```python
from build123d import *

# Parameters (mm, degrees)
SKETCH1_W                                        = 109
SKETCH1_H                                        = 140
BOSS_EXTRUDE1_DEPTH                              = 4
CBORE_FOR_M4_PAN_HEAD_MACHINE_SCREW1_D           = 4.5
CBORE_FOR_M4_PAN_HEAD_MACHINE_SCREW1_CBORE_D     = 9
CBORE_FOR_M4_PAN_HEAD_MACHINE_SCREW1_CBORE_DEPTH = 3.1
SKETCH6_W                                        = 25.091702427
SKETCH6_H                                        = 69.60512686
CUT_EXTRUDE1_DEPTH                               = 89.804560694
SKETCH7_W                                        = 140
SKETCH7_H                                        = 35
BOSS_EXTRUDE2_DEPTH                              = 4
FILLET1_R                                        = 10
BOSS_EXTRUDE3_DEPTH                              = 15
SKETCH9_W                                        = 2
SKETCH9_H                                        = 35
BOSS_EXTRUDE4_DEPTH                              = 140
CUT_EXTRUDE3_DEPTH                               = 101.444014257
SKETCH11_W                                       = 109
SKETCH11_H                                       = 15
CUT_EXTRUDE4_DEPTH                               = 2
FILLET6_R                                        = 5
CUT_EXTRUDE5_REACH                               = 103.198
SKETCH13_W                                       = 4
SKETCH13_H                                       = 73.569558417
CUT_EXTRUDE5_DIRECTION_2_REACH                   = 103.198
SKETCH14_W                                       = 4
SKETCH14_H                                       = 10
BOSS_EXTRUDE5_DEPTH                              = 38.816595147
FILLET9_R                                        = 2.5


with BuildPart() as part:
    # Sketch1 → Boss-Extrude1 (new body)
    with BuildSketch(Plane.XY):
        Rectangle(SKETCH1_W, SKETCH1_H)
    extrude(amount=BOSS_EXTRUDE1_DEPTH)

    # CBORE for M4 Pan Head Machine Screw1 (through all)
    with Locations(Plane.XY.offset(4)):
        with Locations((-19.408297573, 58.521958499), (19.408297573, 58.521958499), (-44.361823025, -9.60512686), (44.559866877, -9.60512686)):
            CounterBoreHole(CBORE_FOR_M4_PAN_HEAD_MACHINE_SCREW1_D / 2, CBORE_FOR_M4_PAN_HEAD_MACHINE_SCREW1_CBORE_D / 2, CBORE_FOR_M4_PAN_HEAD_MACHINE_SCREW1_CBORE_DEPTH)

    # Sketch6 → Cut-Extrude1 (cut, through all)
    with BuildSketch(Plane.XY.offset(4)):
        with Locations((-41.954148786, 35.19743657)):
            Rectangle(SKETCH6_W, SKETCH6_H)
        with Locations((41.954148786, 35.19743657)):
            Rectangle(SKETCH6_W, SKETCH6_H)
    extrude(amount=-CUT_EXTRUDE1_DEPTH, mode=Mode.SUBTRACT)

    # Sketch7 → Boss-Extrude2 (add, through all)
    with BuildSketch(Plane.XY.offset(4)):
        with Locations((0, -52.5)):
            Rectangle(SKETCH7_W, SKETCH7_H)
    extrude(amount=-BOSS_EXTRUDE2_DEPTH)

    # Fillet1
    fillet1_edges = [part.edges().sort_by_distance(p)[0] for p in [
        (-29.408297573, 70, 2),
        (-54.5, 0.39487314, 2),
        (29.408297573, 70, 2),
        (54.5, 0.39487314, 2),
    ]]
    fillet(fillet1_edges, radius=FILLET1_R)

    # Sketch8 → Boss-Extrude3 (add)
    with BuildSketch(Plane.XY.offset(4)):
        Polygon((-70, -35), (-70, -70), (70, -70), (70, -35), (68, -35), (68, -68), (-68, -68), (-68, -35), align=None)
    extrude(amount=BOSS_EXTRUDE3_DEPTH)

    # Sketch9 → Boss-Extrude4 (add, through all)
    with BuildSketch(Plane.ZY.offset(70)):
        with Locations((20, -52.5)):
            Rectangle(SKETCH9_W, SKETCH9_H)
    extrude(amount=-BOSS_EXTRUDE4_DEPTH)

    # Sketch10 → Cut-Extrude3 (cut, through all)
    with BuildSketch(Plane.XY.offset(4)):
        Polygon((-19.408297573, 48.521958499), (-9.408297573, 48.521958499), (-9.408297573, 60), (9.408297573, 60), (9.408297573, 48.521958499), (19.408297573, 48.521958499), (19.408297573, -9.60512686), (34.559866877, -9.60512686), (34.559866877, -19.60512686), (44.5, -19.60512686), (44.5, -60), (-44.5, -60), (-44.5, -19.60512686), (-34.361823025, -19.60512686), (-34.361823025, -9.60512686), (-19.408297573, -9.60512686), align=None)
    extrude(amount=-CUT_EXTRUDE3_DEPTH, mode=Mode.SUBTRACT)

    # Sketch11 → Cut-Extrude4 (cut)
    with BuildSketch(Plane.XY.offset(21)):
        with Locations((0, -42.5)):
            Rectangle(SKETCH11_W, SKETCH11_H)
    extrude(amount=-CUT_EXTRUDE4_DEPTH, mode=Mode.SUBTRACT)

    # Fillet6
    fillet6_edges = [part.edges().sort_by_distance(p)[0] for p in [
        (-54.5, -50, 20),
        (54.5, -50, 20),
        (54.5, -35, 20),
        (-54.5, -35, 20),
    ]]
    fillet(fillet6_edges, radius=FILLET6_R)

    # Cut-Extrude5: up to this face of the body (flat: up to its plane)
    cut_extrude5_end = Plane(part.part.faces().sort_by_distance((-29.408297573, 30.19743657, 2))[0])
    # Sketch13 → Cut-Extrude5 (cut, up to the picked face)
    with BuildSketch(Plane(origin=(0, 0, 0), x_dir=(0, 0, -1), z_dir=(1, 0, 0)), mode=Mode.PRIVATE) as cut_extrude5_sk1:
        with Locations((-2, 37.179652349)):
            Rectangle(SKETCH13_W, SKETCH13_H)
    cut_extrude5_tool1 = split(extrude(cut_extrude5_sk1.sketch, amount=-CUT_EXTRUDE5_REACH, mode=Mode.PRIVATE), bisect_by=cut_extrude5_end, keep=Keep.BOTH, mode=Mode.PRIVATE)
    add(cut_extrude5_tool1.solids().sort_by(Axis((0, 37.179652, 2), (-1, 0, 0)))[0], mode=Mode.SUBTRACT)

    # Cut-Extrude5 direction 2: up to this face of the body (flat: up to its plane)
    cut_extrude5_direction_2_end = Plane(part.part.faces().sort_by_distance((29.408297573, 30.19743657, 2))[0])
    # Sketch13 → Cut-Extrude5 direction 2 (cut, up to the picked face)
    with BuildSketch(Plane(origin=(0, 0, 0), x_dir=(0, 0, -1), z_dir=(1, 0, 0)), mode=Mode.PRIVATE) as cut_extrude5_direction_2_sk1:
        with Locations((-2, 37.179652349)):
            Rectangle(SKETCH13_W, SKETCH13_H)
    cut_extrude5_direction_2_tool1 = split(extrude(cut_extrude5_direction_2_sk1.sketch, amount=CUT_EXTRUDE5_DIRECTION_2_REACH, mode=Mode.PRIVATE), bisect_by=cut_extrude5_direction_2_end, keep=Keep.BOTH, mode=Mode.PRIVATE)
    add(cut_extrude5_direction_2_tool1.solids().sort_by(Axis((0, 37.179652, 2), (1, 0, 0)))[0], mode=Mode.SUBTRACT)

    # Sketch14 → Boss-Extrude5 (add)
    with BuildSketch(Plane.ZY.offset(-19.408297573)):
        with Locations((2, -4.60512686)):
            Rectangle(SKETCH14_W, SKETCH14_H)
    extrude(amount=BOSS_EXTRUDE5_DEPTH)

    # Fillet9
    fillet9_edges = [part.edges().sort_by_distance(p)[0] for p in [
        (34.559866877, -9.60512686, 2),
        (34.559866877, -19.60512686, 2),
        (44.5, -19.60512686, 2),
        (44.5, -60, 2),
        (-44.5, -60, 2),
        (-44.5, -19.60512686, 2),
        (-34.361823025, -19.60512686, 2),
        (-34.361823025, -9.60512686, 2),
    ]]
    fillet(fillet9_edges, radius=FILLET9_R)


solid = part.part
```
Model file for the job. Use its own axes, mm. A direction names the side the tool comes from. Coordinates: 2 decimals unless noted, no trailing zeros. Write each loop counter-clockwise with the first axis right and the second up, starting at its lowest first coordinate (ties: lowest second). Pieces come first, ordered by that corner, then holes. Notation, with made-up numbers: (19, -5.5) - (66, -5.5) arc R30 ccw to (66, 22.5) - close; hole circle Ø2 at (51.25, 77). An arc over 180 degrees is marked (long way). Use a Markdown table: item, result. Add a question column.
Item 1: Two-plate mould, pull along Y, no slides. Class faces 1 (the face through (-51.648, -2.612, 1.972)), 2 (the face through (-39, -19.605, 2)), 3 (the face through (-1, -57, 21)): pulls with the +Y half, pulls with the -Y half, needs draft (parallel to the pull), parting line crosses it, or undercut.
Item 2: 3-axis set-ups, long thin cutter, end or side, ignore diameter. For faces 4 (the face through (-42, -12, 0.9)), 5 (the face through (64, -35, 3)), 6 (the face through (35.27, -18.85, 1.97)): which of +Z, -Z, +X, -X, +Y, -Y reach the whole face in a straight line?
Item 3: Band-saw the part on C-C, the plane x = -13. Write the cut outline in (y, z), and give its area (3 significant figures).
Item 4: Drill centre lines: line 1 along Z through (x, y) = (49, -56.5); line 2 along X through (y, z) = (-44, 16.25); line 3 along Y through (x, z) = (4, 3). Where is each one in solid material? Low to high.
Item 5: Band-saw the part on B-B, the plane z = 2.25. Write the cut outline in (x, y).
Item 6: Band-saw the part on A-A, the plane y = -31.5. Write the cut outline in (x, z).
Item 7: Band-saw the part on D-D, the plane z = 16.75. Write the cut outline in (x, y).
Item 8: Drop flat-ended pins along their axis: pin 1 (1.2 mm diameter, centred on y = -33, z = 1, fed in from +X); pin 2 (14.5 mm diameter, centred on x = 44.56, y = -9.61, fed in from +Z); pin 3 (10 mm diameter, centred on y = -16.5, z = 3.5, fed in from -X); pin 4 (1.5 mm diameter, centred on x = 20.5, y = -11, fed in from +Z). Give the stop position or say it passes through.
A:
| question | item | result |
|---|---|---|
| 1 | face 1 | pulls with the +Y half |
| 1 | face 2 | undercut |
| 1 | face 3 | needs draft |
| 2 | face 4 | +Z |
| 2 | face 5 | +Z, -Z, +X, +Y |
| 2 | face 6 | +Z, -Z |
| 3 | outline | (-70, 0) - (-60, 0) - (-60, 4) - (-68, 4) - (-68, 19) - (-50, 19) - (-50, 21) - (-70, 21) - close; (-9.61, 0) - (0.39, 0) - (0.39, 4) - (-9.61, 4) - close |
| 3 | area | 150 mm² |
| 4 | line 1 | z = 0 to 4, 19 to 21 |
| 4 | line 2 | x = -70 to -68, 68 to 70 |
| 4 | line 3 | y = -70 to -60, -9.61 to 0.39 |
| 5 | outline | (-70, -70) - (70, -70) - (70, -35) - (54.5, -35) - (54.5, -9.61) arc R10 ccw to (44.5, 0.39) - (-44.5, 0.39) arc R10 ccw to (-54.5, -9.61) - (-54.5, -35) - (-70, -35) - close; hole circle Ø9 at (-44.36, -9.61); hole (-44.5, -57.5) arc R2.5 ccw to (-42, -60) - (42, -60) arc R2.5 ccw to (44.5, -57.5) - (44.5, -22.11) arc R2.5 ccw to (42, -19.61) - (37.06, -19.61) arc R2.5 cw to (34.56, -17.11) - (34.56, -12.11) arc R2.5 ccw to (32.06, -9.61) - (-31.86, -9.61) arc R2.5 ccw to (-34.36, -12.11) - (-34.36, -17.11) arc R2.5 cw to (-36.86, -19.61) - (-42, -19.61) arc R2.5 ccw to (-44.5, -22.11) - close; hole circle Ø9 at (44.56, -9.61) |
| 6 | outline | (-54.5, 0) - (-44.5, 0) - (-44.5, 4) - (-54.5, 4) - close; (44.5, 0) - (54.5, 0) - (54.5, 4) - (44.5, 4) - close |
| 7 | outline | (-70, -70) - (70, -70) - (70, -35) - (68, -35) - (68, -68) - (-68, -68) - (-68, -35) - (-70, -35) - close |
| 8 | pin 1 | stops at x = 54.5 |
| 8 | pin 2 | stops at z = 4 |
| 8 | pin 3 | stops at x = -54.5 |
| 8 | pin 4 | passes through |
